Geometry: see drawing. Coordinates: mm, zero at the bounding-box minimum. A direction names the side the tool comes from. Round coordinates to 2 decimals unless told otherwise and drop trailing zeros. Order: outer loops, then holes, each group sorted by start corner. A loop starts at its lowest first (then second) coordinate and runs counter-clockwise, first axis right, second up. Notation, with made-up numbers: (78.25, 41) -> (108.25, 41) arc R22 ccw to (108.25, 77) -> close; hole circle Ø10 at (52.25, 35). An arc over 180 degrees is marked (long way). Put each result on its own line as item: value.
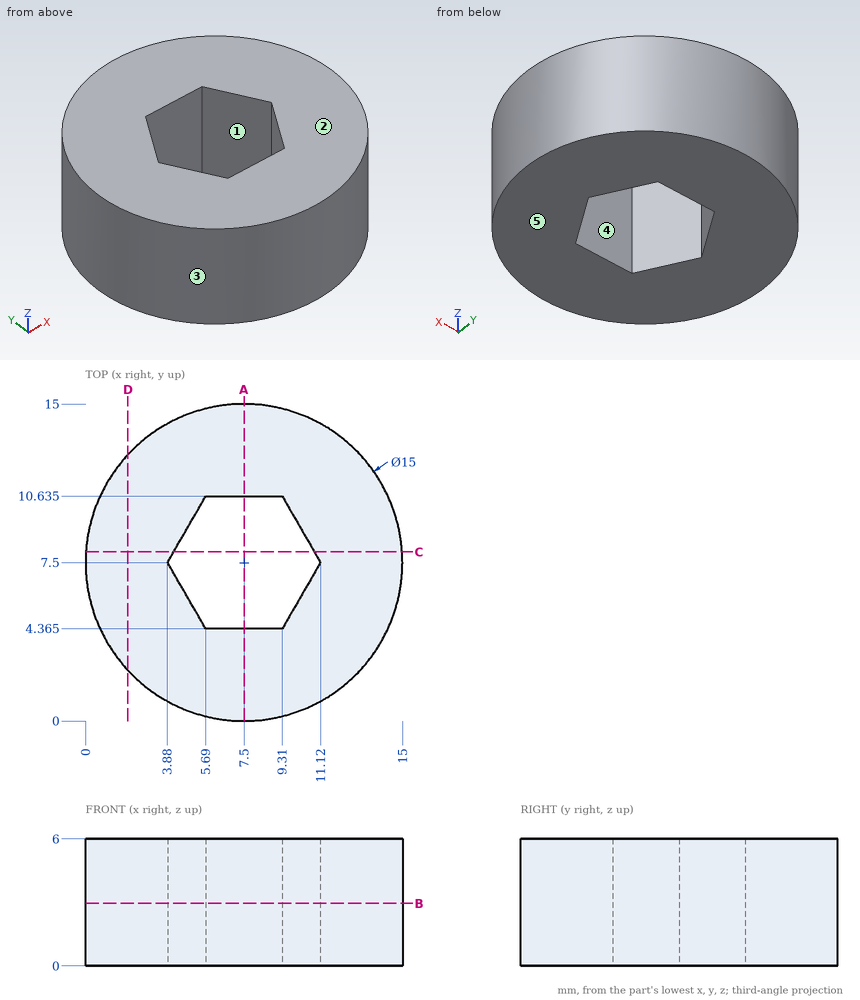
1. Material intervals for probe 1 along Y at (x, z) = (8.25, 4.8) (1 decimal); probe 2 along Y at (x, z) = (10.75, 1.25); probe 3 along X at (y, z) = (9.75, 4.6) (1 decimal), sorted ascending.
Ans:
probe 1: 0 to 4.4, 10.6 to 15
probe 2: 0.74 to 6.86, 8.14 to 14.26
probe 3: 0.3 to 5.2, 9.8 to 14.7
2. Cut plane C-C on y = 8. Return loops of the section in (x, z).
Ans:
outline: (0.02, 0) -> (4.17, 0) -> (4.17, 6) -> (0.02, 6) -> close; (10.83, 0) -> (14.98, 0) -> (14.98, 6) -> (10.83, 6) -> close
3. Set-up query: the marked faces 1 and 2. Return all of +Z, -Z, +X, -X, +Y, -Y with unobstructed straight access to the full face (end or side cutting, diameter ignored); none if empty.
Ans:
face 1: +Z, -Z
face 2: +Z, +X, -X, +Y, -Y
4. Cut plane D-D on x = 2. Return loops of the section in (y, z), and give its area (3 significant figures).
Ans:
outline: (2.4, 0) -> (12.6, 0) -> (12.6, 6) -> (2.4, 6) -> close
area: 61.2 mm²
5. Cut plane A-A on x = 7.5. Return loops of the section in (y, z) (1 decimal), and give its area (3 significant figures).
Ans:
outline: (0, 0) -> (4.4, 0) -> (4.4, 6) -> (0, 6) -> close; (10.6, 0) -> (15, 0) -> (15, 6) -> (10.6, 6) -> close
area: 52.4 mm²
6. Contact query for flat-ended pins moving along their axis: P1, Ø1, axis at x = 8.5, z = 2.5, coming from the +Y side; P2, Ø1.5, axis at x = 11.5, z = 2, coming from the -Y side. Output: stop coordinate, or through.
Ans:
P1: y = 14.98
P2: y = 0.74
7. Draft query along X for the marked faces 3, 4 and 5. Return one class per face: +X half, -X half, draft (parallel to the pull), parting line (faces both ways), or undercut.
Ans:
face 3: parting line
face 4: undercut
face 5: draft
8. Cut plane B-B on z = 2.95. Return loops of the section in (x, y) (1 decimal), and give its area (3 significant figures).
Ans:
outline: circle Ø15 at (7.5, 7.5); hole (3.9, 7.5) -> (5.7, 4.4) -> (9.3, 4.4) -> (11.1, 7.5) -> (9.3, 10.6) -> (5.7, 10.6) -> close
area: 143 mm²
